CAD build for the part. Positions are in the model's coordinates, mm. Face numbers are marked on the shaded views. A direction names the side the tool comes from. Give positions to 0.01 mm unless a question says otherwise; leave off trailing zeros. Order: outer loops, then holes, each group sorted by start corner. A loop starts at its lowest first (then second) coordinate and runs counter-clockwise, first axis right, second up.
Item 1: Band-saw the part on B-B on y = 5. Give the cut face in (x, z), plus the area to 3 significant figures.
Item 2: Which spindle directions (+Z, -Z, +X, -X, +Y, -Y) get a long thin tool onto all of the face, cutting with end or side? Do the marked faces 4 and 5. Say none if no direction does.
Item 3: Flat gauge pin, fed straight in: P1, Ø3, axis at y = 3.5, z = 7.5, coming from the +X side. Where does the tip first touch, or does it go through?
Item 4: Wall check: L1, parallel to Z at x = -75, y = 5.5; L2, parallel to Z at x = -80.5, y = 7; L3, parallel to Z at x = -58.5, y = 3.75. Give the ranges that are in metal, low to high.
Item 5: Band-saw the part on D-D on x = -73. Give the cut face in (y, z), plus the area to 3 significant figures.
Item 6: Band-saw the part on A-A on x = -59. Give the cut face in (y, z).
Item 7: Two-plate mould, pull along Z, no slides. Class the marked faces 1, 2 and 3: released by +Z, released by -Z, zero draft, split by the parting line, or undercut.
Item 8: Band-saw the part on C-C on z = 57. Give the cut face in (x, y).
```python
from build123d import *

# Parameters (mm, degrees)
BOSS_EXTRU_3_DEPTH = 10


with BuildPart() as part:
    # Esquisse5 → Boss.-Extru.3 (new body)
    with BuildSketch(Plane(origin=(0, 0, 0), x_dir=(1, 0, 0), z_dir=(0, 1, 0))):
        Polygon((-57, 52), (-57, 62), (-87, 62), (-87, -62), (-57, -62), (-57, -52), (-77, -52), (-77, 52), align=None)
        with BuildLine():
            Line((-81, 59.1), (-63, 59.1))
            ThreePointArc((-63, 59.1), (-60.9, 57), (-63, 54.9))
            Line((-63, 54.9), (-81, 54.9))
            ThreePointArc((-81, 54.9), (-83.1, 57), (-81, 59.1))
        make_face(mode=Mode.SUBTRACT)
        with BuildLine():
            Line((-81, -59.1), (-63, -59.1))
            ThreePointArc((-63, -59.1), (-60.9, -57), (-63, -54.9))
            Line((-63, -54.9), (-81, -54.9))
            ThreePointArc((-81, -54.9), (-83.1, -57), (-81, -59.1))
        make_face(mode=Mode.SUBTRACT)
    extrude(amount=BOSS_EXTRU_3_DEPTH)


solid = part.part
```
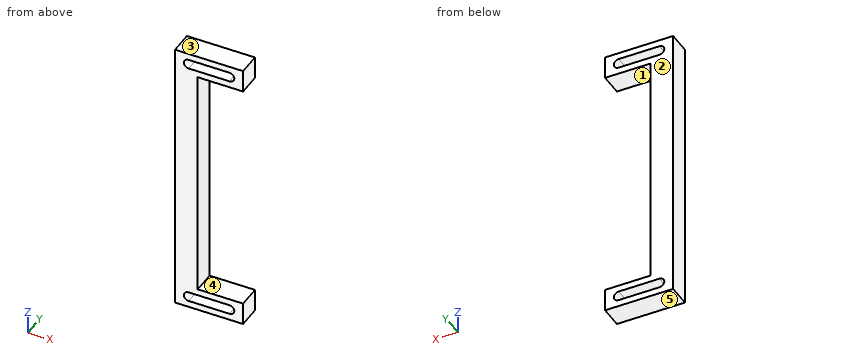
The answers:
1. outline: (-87, -62) - (-57, -62) - (-57, -52) - (-77, -52) - (-77, 52) - (-57, 52) - (-57, 62) - (-87, 62) - close; hole (-81, -59.1) - (-63, -59.1) arc R2.1 ccw to (-63, -54.9) - (-81, -54.9) arc R2.1 ccw to start; hole (-81, 54.9) - (-63, 54.9) arc R2.1 ccw to (-63, 59.1) - (-81, 59.1) arc R2.1 ccw to start
1. area: 1,460 mm2
2. face 4: +X, +Y, -Y
2. face 5: -Z, +X, -X, +Y, -Y
3. P1: stops at x = -77
4. L1: z = -62 to -59.1, -54.9 to -52, 52 to 54.9, 59.1 to 62
4. L2: z = -62 to -59.1, -54.9 to 54.9, 59.1 to 62
4. L3: z = -62 to -52, 52 to 62
5. outline: (0, -62) - (10, -62) - (10, -59.1) - (0, -59.1) - close; (0, -54.9) - (10, -54.9) - (10, -52) - (0, -52) - close; (0, 52) - (10, 52) - (10, 54.9) - (0, 54.9) - close; (0, 59.1) - (10, 59.1) - (10, 62) - (0, 62) - close
5. area: 116 mm2
6. outline: (0, -62) - (10, -62) - (10, -52) - (0, -52) - close; (0, 52) - (10, 52) - (10, 62) - (0, 62) - close
7. face 1: undercut
7. face 2: zero draft
7. face 3: released by +Z
8. outline: (-87, 0) - (-83.1, 0) - (-83.1, 10) - (-87, 10) - close; (-60.9, 0) - (-57, 0) - (-57, 10) - (-60.9, 10) - close
